from build123d import *

# Parameters (mm, degrees)
SKETCH1_W          = 204
SKETCH1_H          = 300
BASE_FLANGE1_DEPTH = 1
EDGE_FLANGE1_DEPTH = 300


# Sheet-metal steps are written as plain solids
with BuildPart() as part:
    # Sketch1 → Base-Flange1 (new body)
    with BuildSketch(Plane.XY):
        Rectangle(SKETCH1_W, SKETCH1_H)
    extrude(amount=-BASE_FLANGE1_DEPTH)

    # Edge-Flange1 section (across the edge) → Edge-Flange1 (add)
    with BuildSketch(Plane(origin=(103, 150, -1), x_dir=(-1, 0, 0), z_dir=(0, -1, 0))):
        with BuildLine():
            Line((-1, 1), (-1, 9))
            Line((-1, 9), (0, 9))
            Line((0, 9), (0, 1))
            ThreePointArc((0, 1), (0.292893219, 0.292893219), (1, 0))
            Line((1, 0), (1, -1))
            ThreePointArc((1, -1), (-0.414213562, -0.414213562), (-1, 1))
        make_face()
    edge_flange1 = extrude(amount=EDGE_FLANGE1_DEPTH)

    # Mirror1: Edge-Flange1 across plane
    add(edge_flange1.mirror(Plane(origin=(0, 0, 0), x_dir=(0, 0, 1), z_dir=(1, 0, 0))))


solid = part.part
Build history of the part. All positions in model axes, mm. A direction names the side the tool comes from. Give positions to 0.01 mm unless a question says otherwise; leave off trailing zeros. Order: outer loops, then holes, each group sorted by start corner. A loop starts at its lowest first (then second) coordinate and runs counter-clockwise, first axis right, second up. Notation, with made-up numbers: M 22,-4 L 76,-4 A19 cw 76,12 Z; hole C -28.5,36 d4. An arc over 180 degrees is marked long. Use one line per item in the form item = value.
Q1. Slice it at A-A, the plane z = -4.5. Write the cut outline in (x, y).
Conclusion:
outline = M -104,-150 L -103,-150 L -103,150 L -104,150 Z; M 103,-150 L 104,-150 L 104,150 L 103,150 Z
Q2. Slice it at C-C, the plane x = 33. Write the cut outline in (y, z), and give its area (3 significant figures).
Conclusion:
outline = M -150,-1 L 150,-1 L 150,0 L -150,0 Z
area = 300 mm2
Q3. Which spindle directions (+Z, -Z, +X, -X, +Y, -Y) get a long thin tool onto all of the face, cutting with end or side? Do faces 5 (the flat face through (0.5, -150, -0.6)), 6 (the flat face through (-1, 2, -1)). Say none if no direction does.
Conclusion:
face_5 = +Z, -Z, +X, -X, -Y
face_6 = -Z, +Y, -Y
Q4. Pull direction X, two halves, no side cores. Call faces 1 (the flat face through (0.5, 150, -0.6)), 2 (the flat face through (103, 2, -6)), 3 (the flat face through (-104, 2, -6)), 4 (the flat face through (104, 2, -6)): released by +X, released by -X, zero draft, split by the parting line, or undercut.
Conclusion:
face_1 = zero draft
face_2 = undercut
face_3 = released by -X
face_4 = released by +X
Q5. Wall check: probe 1 along X at (y, z) = (49.5, -9.25); probe 2 along Z at (x, y) = (-25.5, 128). Give the ranges that are in metal, low to high.
Conclusion:
probe_1 = -104 to -103, 103 to 104
probe_2 = -1 to 0
Q6. Slice it at B-B, the plane y = -86. Write the cut outline in (x, z).
Conclusion:
outline = M -104,-10 L -103,-10 L -103,-2 A1 cw -102,-1 L 102,-1 A1 cw 103,-2 L 103,-10 L 104,-10 L 104,-2 A2 ccw 102,0 L -102,0 A2 ccw -104,-2 Z
